For this review, use the dimensioned drawing (mm, ordinates from the lowest corner) and the shaded views. Round coordinates to 2 decimals unless told otherwise and drop trailing zeros. Loops run counter-clockwise (first coordinate to the right, second up) from the corner with the lowest first, then second, coordinate; pieces in that order, holes last. Notation, with made-up numbers: M 7.5,8.5 L 30.5,8.5 A24 cw 30.5,43.5 Z; hole C 74,65.5 d7. An arc over 180 degrees is marked long. One line per item, written item: value. Start each with the question number.
Item 1: We need section B-B (y = 87). Write out the cut boundary in (x, z), then the cut area to 3 significant figures.
Item 2: For line 1 along Y through (x, z) = (2.8, 13); line 2 along Z through (x, y) = (1.3, 52); line 3 along X through (y, z) = (76.5, 8.5), list the stretches that pass through material, from the lowest coordinate up.
Item 3: We need section A-A (z = 2). Write out the cut boundary in (x, y), then the cut area to 3 significant figures.
Item 4: We need section C-C (y = 66). Write out the cut boundary in (x, z).
Item 5: Clearance check with flat-ended pins moving along their axes: pin 1 (1 mm diameter, centred on y = 77, z = 4.5, fed in from -X); pin 2 (1.5 mm diameter, centred on x = 2, z = 10, fed in from +Y). State where each tip first meets the part, or that it passes through.
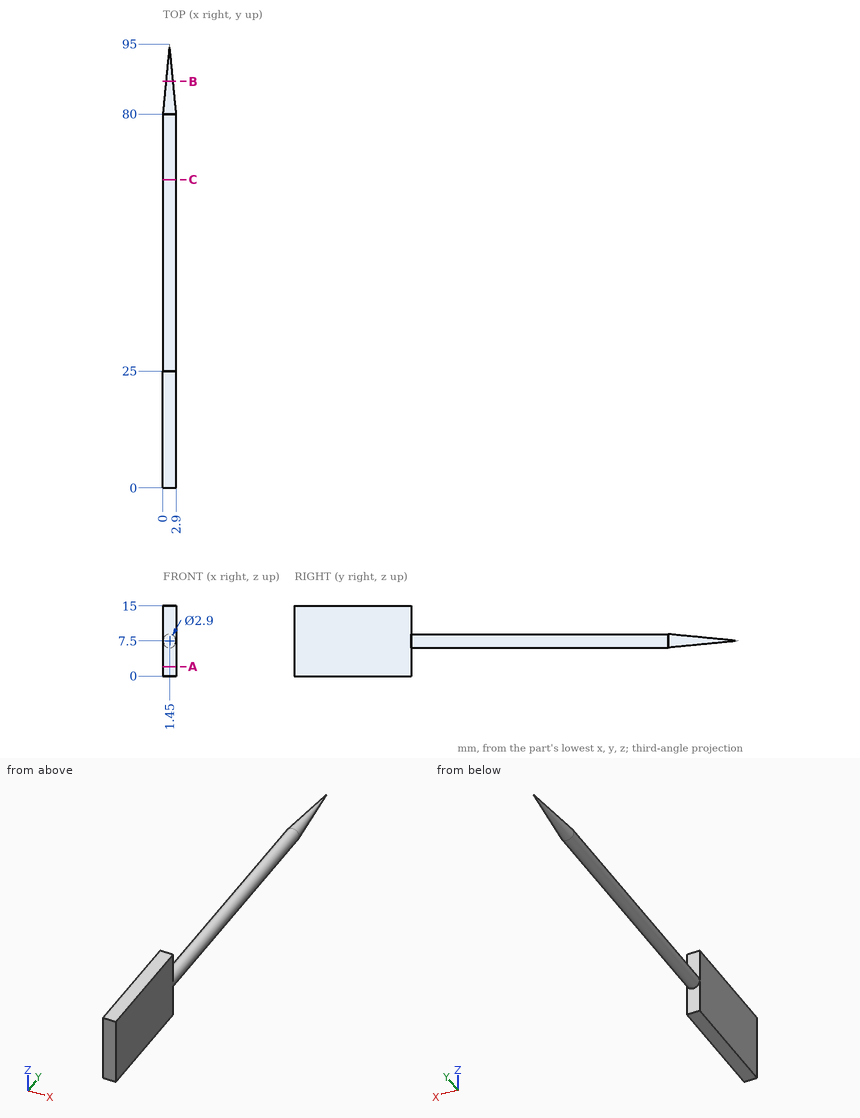
A:
1. outline: C 1.45,7.5 d1.55
1. area: 1.88 mm2
2. line 1: 0 to 25
2. line 2: 6.06 to 8.94
2. line 3: 0.4 to 2.5
3. outline: M 0,0 L 2.9,0 L 2.9,25 L 0,25 Z
3. area: 72.5 mm2
4. outline: C 1.45,7.5 d2.9
5. pin 1: through
5. pin 2: y = 25
